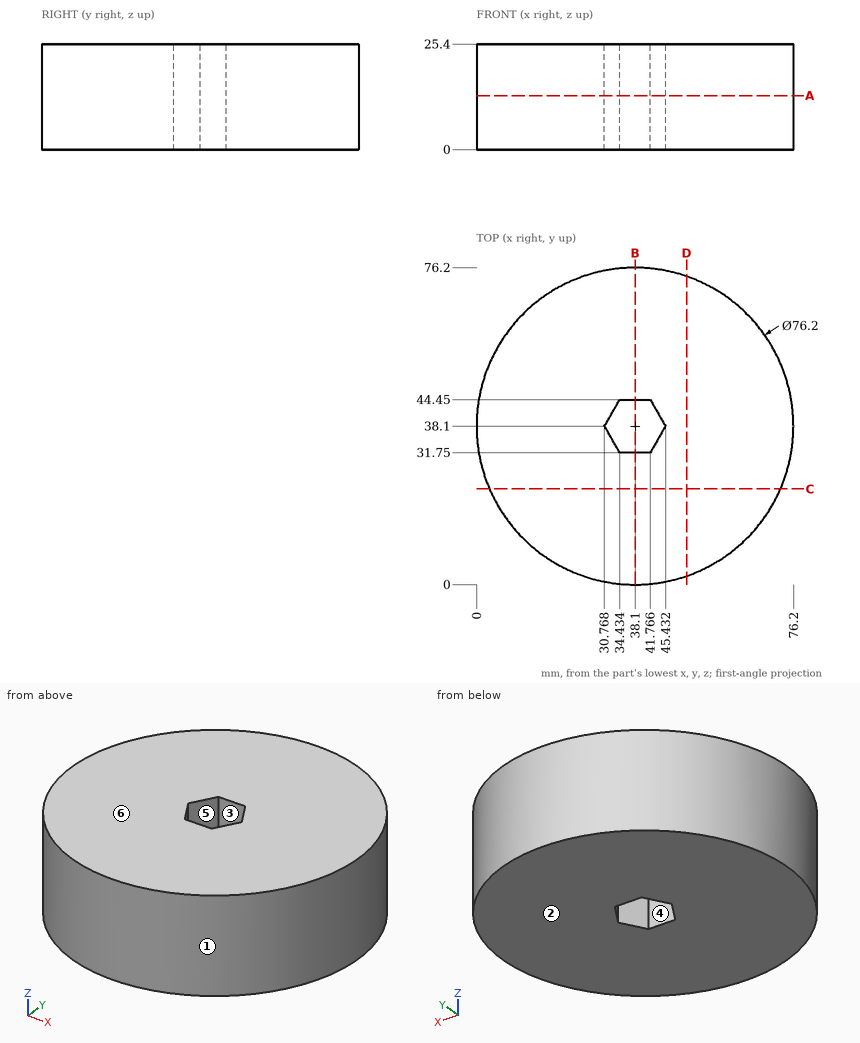
Part print with two shaded views. Sizes in mm from the minimum x, y, z corner. A direction names the side the tool comes from. Round coordinates to 2 decimals unless told otherwise and drop trailing zeros. Loops run counter-clockwise (first coordinate to the right, second up) from the corner with the lowest first, then second, coordinate; pieces in that order, holes last.
Item 1: Saw through at A-A (z = 13). List the corners of the cut face in (x, y), then the cut area to 3 significant figures.
Item 2: Two-plate mould, pull along X, no slides. Class the marked faces 1, 2, 3 and 4: released by +X, released by -X, zero draft, split by the parting line, or undercut.
Item 3: Drill centre lines: line 1 along X through (y, z) = (37, 9.75) (1 decimal); line 2 along Y through (x, z) = (31.5, 2.75) (1 decimal); line 3 along Y through (x, z) = (43, 12.5) (1 decimal). Where is each one in solid material? Low to high.
Item 4: Saw through at C-C (y = 23). List the corners of the cut face in (x, z), then the cut area to 3 significant figures.
Item 5: Pin check, flat tips, straight feed: P1, Ø4, axis at y = 42.5, z = 15, coming from the -X side; P2, Ø8, axis at x = 41.5, z = 7.5, coming from the -Y side; P3, Ø8, axis at y = 47, z = 13.5, coming from the +X side. Stop position of each tip, or through.
Item 6: Saw through at D-D (x = 50.5). List the corners of the cut face in (y, z).
Item 7: Saw through at B-B (x = 38.1). List the corners of the cut face in (y, z).
Item 8: Which spindle directions (+Z, -Z, +X, -X, +Y, -Y) get a long thin tool onto all of the face, cutting with end or side? Do the marked faces 5 and 6. Say none if no direction does.
Worked answers:
1. outline: circle Ø76.2 at (38.1, 38.1); hole (30.77, 38.1) - (34.43, 31.75) - (41.77, 31.75) - (45.43, 38.1) - (41.77, 44.45) - (34.43, 44.45) - close
1. area: 4,420 mm2
2. face 1: split by the parting line
2. face 2: zero draft
2. face 3: undercut
2. face 4: undercut
3. line 1: x = 0 to 31.4, 44.8 to 76.2
3. line 2: y = 0.6 to 36.8, 39.4 to 75.6
3. line 3: y = 0.3 to 33.9, 42.3 to 75.9
4. outline: (3.12, 0) - (73.08, 0) - (73.08, 25.4) - (3.12, 25.4) - close
4. area: 1,780 mm2
5. P1: stops at x = 0.08
5. P2: stops at y = 0
5. P3: stops at x = 75.88
6. outline: (2.07, 0) - (74.13, 0) - (74.13, 25.4) - (2.07, 25.4) - close
7. outline: (0, 0) - (31.75, 0) - (31.75, 25.4) - (0, 25.4) - close; (44.45, 0) - (76.2, 0) - (76.2, 25.4) - (44.45, 25.4) - close
8. face 5: +Z, -Z
8. face 6: +Z, +X, -X, +Y, -Y
